For this review, take the finished solid that the model builds, in its own axes (mm). Face numbers are marked on the shaded views. A direction names the side the tool comes from. Give positions to 0.01 mm unless a question says otherwise; leave off trailing zeros. Write each loop counter-clockwise with the first axis right and the second up, starting at its lowest first coordinate (ties: lowest second). Pieces come first, ordered by that corner, then holes. Notation, with made-up numbers: M 19,32 L 48,32 A19 cw 48,64 Z; hole C 9.5,-20 d4. An arc over 180 degrees is marked long. Write item = value, one per line.
```python
from build123d import *

# Parameters (mm, degrees)
F1_DEPTH    = 48
F2_DEPTH    = 10
F3_R        = 6
F4_T1_DEPTH = 30
F5_W        = 28
F5_H        = 5
F6_DEPTH    = 5
F5_R        = 6
F7_DEPTH    = 3
F8_DEPTH    = 30.001


# Not quite as in the source:
# - a fillet or chamfer that OpenCascade refuses, or shapes differently, is made with other operations: its cross-section is extruded or revolved along the edge and cut away or added


with BuildPart() as f1:
    # F0 (on Top) → F1 (new body)
    with BuildSketch(Plane.XY):
        Polygon((31, -6), (31, 24), (21, 24), (21, 4), (-21, 4), (-21, 24), (-31, 24), (-31, -6), align=None)
    extrude(amount=F1_DEPTH)

    # F0 (on Top) → F2 (join)
    with BuildSketch(Plane.XY):
        Polygon((-46, -24), (46, -24), (46, 24), (31, 24), (31, -6), (-31, -6), (-31, 24), (-46, 24), align=None)
        Polygon((31, -6), (31, 24), (21, 24), (21, 4), (-21, 4), (-21, 24), (-31, 24), (-31, -6), align=None)
    extrude(amount=F2_DEPTH)

    # F3
    f3_edges = [f1.edges().sort_by_distance(p)[0] for p in [
        (-46, -24, 5),
        (46, -24, 5),
    ]]
    fillet(f3_edges, radius=F3_R)

    # F4: fillet of radius 25 on 2 edges, made by hand

    # F4_s2 → F4_t1 (join)
    with BuildSketch(Plane.XZ.offset(-24)):
        with BuildLine():
            ThreePointArc((-46, 10), (-35.0834993366, 19.2198145372), (-31, 32.9128784748))
            Line((-31, 32.9128784748), (-31, 10))
            Line((-31, 10), (-46, 10))
        make_face()
        with BuildLine():
            ThreePointArc((46, 10), (35.0834993366, 19.2198145372), (31, 32.9128784748))
            Line((31, 32.9128784748), (31, 10))
            Line((31, 10), (46, 10))
        make_face()
    extrude(amount=F4_T1_DEPTH)

    # F5 (on face) → F6 (join)
    with BuildSketch(Plane.XZ.offset(6)):
        with Locations((0, 12.5)):
            Rectangle(F5_W, F5_H)
    extrude(amount=F6_DEPTH)

    # F5 (on face) → F7 (join)
    with BuildSketch(Plane.XZ.offset(6)):
        with BuildLine():
            Line((14, 15), (14, 29))
            ThreePointArc((14, 29), (0, 43), (-14, 29))
            Line((-14, 29), (-14, 15))
            Line((-14, 15), (14, 15))
        make_face()
        with Locations((0, 29)):
            Circle(F5_R, mode=Mode.SUBTRACT)
    extrude(amount=F7_DEPTH)

    # F8 (cut, through all): a face of the model
    f8_faces = [f1.faces().sort_by_distance(p)[0] for p in [
        (0, -6, 29),
    ]]
    extrude(f8_faces, amount=-F8_DEPTH, mode=Mode.SUBTRACT)


solid = f1.part
```
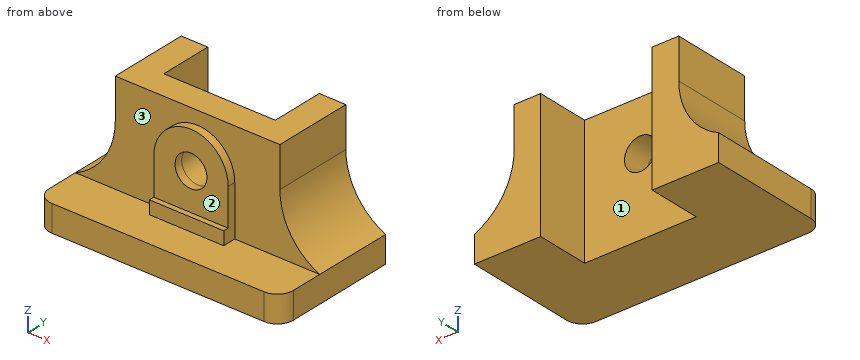
1. We need section B-B, the plane y = 18. Write out the cut boundary in (x, z).
Responses:
outline = M -46,0 L -21,0 L -21,48 L -31,48 L -31,32.91 A25 cw -46,10 Z; M 21,0 L 46,0 L 46,10 A25 cw 31,32.91 L 31,48 L 21,48 Z
2. We need section A-A, the plane x = 0. Write out the cut boundary in (y, z), then the cut area to 3 significant figures.
Responses:
outline = M -24,0 L 4,0 L 4,23 L -9,23 L -9,15 L -11,15 L -11,10 L -24,10 Z; M -9,35 L 4,35 L 4,48 L -6,48 L -6,43 L -9,43 Z
area = 613 mm2
3. Insertion check: P1, Ø12, axis at y = 14.5, z = 38.5, coming from the +X side; P2, Ø4, axis at y = -9.5, z = 16, coming from the +X side; P3, Ø10, axis at x = 18, z = 33.5, coming from the -Y side. Each pin has a flat end and moves straight along its axis. Give the tip position at first contact, or say it passes through.
Responses:
P1 = 31
P2 = 14
P3 = -9
4. We need section D-D, the plane x = 26. Write out the cut boundary in (y, z), then the cut area to 3 significant figures.
Responses:
outline = M -24,0 L 24,0 L 24,48 L -6,48 L -6,10 L -24,10 Z
area = 1,620 mm2
5. For line 1 along Z through (x, y) = (0, 1.5); line 2 along Z through (x, y) = (0, -7.25); line 3 along Z through (x, y) = (-2.5, -13.5), list the stretches that pass through material, from the lowest coordinate up. Write a range as from..to.
Responses:
line_1 = 0..23, 35..48
line_2 = 0..23, 35..43
line_3 = 0..10
6. Machinability: for the marked faces 1, 2 and 3, which of the approach directions +Z, -Z, +X, -X, +Y, -Y give a long, thin tool a straight path to every point of the face, cutting with its end or side? Answer none if there is none.
Responses:
face_1 = +Z, -Z, +Y
face_2 = +Z, +X, -X, -Y
face_3 = +Z, -Y
7. We need section C-C, the plane z = 44. Write out the cut boundary in (x, y).
Responses:
outline = M -31,-6 L 31,-6 L 31,24 L 21,24 L 21,4 L -21,4 L -21,24 L -31,24 Z
